The model under review builds one solid part; all positions refer to its coordinate system, in mm. A direction names the side the tool comes from. Coordinates: 2 decimals unless noted, no trailing zeros. Write each loop counter-clockwise with the first axis right and the second up, starting at its lowest first coordinate (ties: lowest second). Pieces come first, ordered by that corner, then holes. Notation, with made-up numbers: (68, -11.75) - (107, -11.75) arc R19 cw to (107, -4.75) - close; hole circle Ø9 at (44.5, 3.5). An arc over 180 degrees is marked (long way). Put each result on its own line as item: value. Start each with the question number.
Item 1: Mouldability with a two-part tool opening along X and no side actions: class faces 1 (the face through (107.418, 4.93, -38.356)), 2 (the face through (30.89, 4.93, -0.52)), 3 (the face through (198.212, 45, 0)), 4 (the face through (228, 38, 0)) as pulls with the +X half, pulls with the -X half, needs draft (parallel to the pull), parting line crosses it, or undercut.
Item 2: Machinability: for faces 5 (the face through (103.92, 45.99, 0.1)), 6 (the face through (98.212, 22, 0)), 7 (the face through (111.926, 5, 0)), 8 (the face through (103, 54, 9)), which of the approach directions +Z, -Z, +X, -X, +Y, -Y give a long, thin tool a straight path to every point of the face, cutting with its end or side? Answer none if there is none.
Item 3: For pin 1 (16 mm diameter, centred on x = 250.5, z = -2, fed in from -Y); pin 2 (7 mm diameter, centred on y = 20.5, z = -1.5, fed in from -X); pin 3 (6 mm diameter, centred on y = 40.5, z = 16, fed in from -X), all flat-tipped, find the tip position at first contact; note any pin that passes through.
Item 4: Consider section B-B on y = 23. Give the boundary of the cut face in (x, z), then the cut area to 3 significant figures.
Item 5: Consider section A-A on z = 0. State how many separate pieces and enclosed holes the cut face has, then the cut area to 3 significant figures.
Item 6: To check wall thickness, follow L1, parallel to X at y = 54, z = 0; L2, parallel to X at y = 68, z = 3.5; L3, parallel to Z at x = 172, y = 76. State the ranges of each line that lie inside material, in increasing order. Write a range as [from, to].
```python
from build123d import *

# Parameters (mm, degrees)
SKETCH1_R           = 4
BOSS_EXTRUDE1_DEPTH = 10
BOSS_EXTRUDE2_DEPTH = 9
BOSS_EXTRUDE3_DEPTH = 16
SKETCH3_R           = 4.5
CUT_EXTRUDE1_DEPTH  = 274.856521232
FILLET5_R           = 2


with BuildPart() as part:
    # Sketch1 → Boss-Extrude1 (new body)
    with BuildSketch(Plane(origin=(0, 0, 0), x_dir=(1, 0, 0), z_dir=(0, 1, 0))):
        with BuildLine():
            Line((23.211917272, 9.284766909), (98.211917272, 39.284766909))
            ThreePointArc((98.211917272, 39.284766909), (107.532112129, 38.280672305), (111.925824036, 30))
            Line((111.925824036, 30), (111.925824036, -30))
            ThreePointArc((111.925824036, -30), (107.532112129, -38.280672305), (98.211917272, -39.284766909))
            Line((98.211917272, -39.284766909), (23.211917272, -9.284766909))
            ThreePointArc((23.211917272, -9.284766909), (16.925824036, 0), (23.211917272, 9.284766909))
        make_face()
        with Locations(Location((26.925824036, 0, 0), (0, 0, 270))):
            Circle(SKETCH1_R, mode=Mode.SUBTRACT)
        with Locations(Location((101.925824036, 30, 0), (0, 0, 270))):
            Circle(SKETCH1_R, mode=Mode.SUBTRACT)
        with Locations(Location((101.925824036, -30, 0), (0, 0, 270))):
            Circle(SKETCH1_R, mode=Mode.SUBTRACT)
    extrude(amount=BOSS_EXTRUDE1_DEPTH)

    # Sketch2 → Boss-Extrude2 (add, symmetric)
    with BuildSketch(Plane.XY):
        with BuildLine():
            Line((98.211917272, 10), (98.211917272, 32))
            ThreePointArc((98.211917272, 32), (104.069781648, 46.142135624), (118.211917272, 52))
            Line((118.211917272, 52), (198.211917272, 52))
            Line((198.211917272, 52), (198.211917272, 82))
            Line((198.211917272, 82), (93.211917272, 82))
            ThreePointArc((93.211917272, 82), (57.856578213, 67.355339059), (43.211917272, 32))
            Line((43.211917272, 32), (43.211917272, 10))
            Line((43.211917272, 10), (98.211917272, 10))
        make_face()
    extrude(amount=BOSS_EXTRUDE2_DEPTH, both=True)

    # Sketch2_4 → Boss-Extrude3 (add, symmetric)
    with BuildSketch(Plane.XY):
        with BuildLine():
            Line((258.211917272, 82), (198.211917272, 82))
            Line((198.211917272, 82), (198.211917272, 52))
            Line((198.211917272, 52), (198.211917272, 38))
            Line((198.211917272, 38), (258.211917272, 38))
            Line((258.211917272, 38), (258.211917272, 59))
            Line((258.211917272, 59), (238.178546819, 59))
            ThreePointArc((238.178546819, 59), (208.211917272, 60), (238.178546819, 61))
            Line((238.178546819, 61), (258.211917272, 61))
            Line((258.211917272, 61), (258.211917272, 82))
        make_face()
    extrude(amount=BOSS_EXTRUDE3_DEPTH, both=True)

    # Sketch3 → Cut-Extrude1 (cut, through all)
    with BuildSketch(Plane(origin=(0, 82, 0), x_dir=(1, 0, 0), z_dir=(0, 1, 0))):
        with Locations(Location((248.211917272, 0, 0), (0, 0, 270))):
            Circle(SKETCH3_R)
    extrude(amount=-CUT_EXTRUDE1_DEPTH, mode=Mode.SUBTRACT)

    # Fillet5
    fillet5_edges = [part.edges().sort_by_distance(p)[0] for p in [
        (98.211917272, 21, -9),
        (98.211917272, 10, 0),
        (104.069781648, 46.142135624, -9),
        (158.211917272, 52, 9),
        (198.211917272, 67, 9),
        (198.211917272, 52, 0),
        (145.711917272, 82, 9),
        (57.856578213, 67.355339059, 9),
        (43.211917272, 21, 9),
        (70.711917272, 10, 9),
        (43.211917272, 10, 0),
        (98.211917272, 21, 9),
        (104.069781648, 46.142135624, 9),
        (70.711917272, 10, -9),
        (43.211917272, 21, -9),
        (57.856578213, 67.355339059, -9),
        (145.711917272, 82, -9),
        (198.211917272, 67, -9),
        (158.211917272, 52, -9),
        (198.211917272, 82, -12.5),
        (198.211917272, 82, 12.5),
    ]]
    fillet(fillet5_edges, radius=FILLET5_R)


solid = part.part
```
Report:
1. face 1: parting line crosses it
1. face 2: undercut
1. face 3: undercut
1. face 4: needs draft
2. face 5: +Z, -Z
2. face 6: +Z, -Z, +X
2. face 7: +Z, -Z, +X, -Y
2. face 8: +Z, -X, +Y
3. pin 1: y = 38
3. pin 2: x = 43.21
3. pin 3: x = 198.21
4. outline: (43.21, -7) arc R2 ccw to (45.21, -9) - (96.21, -9) arc R2 ccw to (98.21, -7) - (98.21, 7) arc R2 ccw to (96.21, 9) - (45.21, 9) arc R2 ccw to (43.21, 7) - close
4. area: 987 mm²
5. separate pieces: 4
5. enclosed holes: 0
5. area: 8,900 mm²
6. L1: [48.31, 209.46], [236.96, 243.71], [252.71, 258.21]
6. L2: [58.51, 210.52], [235.9, 245.38], [251.04, 258.21]
6. L3: [-9, 9]
